```python
from build123d import *

# Parameters (mm, degrees)
BOX001_W        = 35
BOX001_H        = 47
BOX001_DEPTH    = 4
SKETCH006_W     = 6.802042
SKETCH006_H     = 4
PAD003_DEPTH    = 14
SKETCH007_R     = 1.647159
SKETCH007_R_2   = 1.531135
POCKET003_DEPTH = 7
PAD004_DEPTH    = 4
SKETCH009_R     = 4.5
SKETCH009_R_2   = 1.7
POCKET004_DEPTH = 4


with BuildPart() as part:
    # Box001 → Box001 (new body)
    with BuildSketch(Plane(origin=(-11, -31, -17), x_dir=(1, 0, 0), z_dir=(0, 0, 1))):
        with Locations((17.5, 23.5)):
            Rectangle(BOX001_W, BOX001_H)
    extrude(amount=BOX001_DEPTH)

    # Sketch006 → Pad003 (new body)
    with BuildSketch(Plane(origin=(-11, -31, -17), x_dir=(1, 0, 0), z_dir=(0, 0, -1))):
        with Locations((9.901021, -9.91944)):
            Rectangle(SKETCH006_W, SKETCH006_H)
        with Locations((9.901021, -37.91944)):
            Rectangle(SKETCH006_W, SKETCH006_H)
    extrude(amount=PAD003_DEPTH)

    # Sketch007 → Pocket003 (cut)
    with BuildSketch(Plane(origin=(2.302042, -31, -17), x_dir=(0, 1, 0), z_dir=(1, 0, 0))):
        with Locations((9.935232, -7.037912)):
            Circle(SKETCH007_R)
        with Locations((37.888477, -7.037912)):
            Circle(SKETCH007_R_2)
    extrude(amount=-POCKET003_DEPTH, mode=Mode.SUBTRACT)

    # Sketch008 → Pad004 (new body)
    with BuildSketch(Plane(origin=(-11, -31, -17), x_dir=(1, 0, 0), z_dir=(0, 0, -1))):
        with BuildLine():
            ThreePointArc((35, -34.9498), (43.145898, -23.9498), (35, -12.9498))
            Line((35, -12.9498), (35, -34.9498))
        make_face()
        with BuildLine():
            ThreePointArc((0, -12.9498), (-8.145898, -23.9498), (0, -34.9498))
            Line((0, -12.9498), (0, -34.9498))
        make_face()
    extrude(amount=-PAD004_DEPTH)

    # Sketch009 → Pocket004 (cut)
    with BuildSketch(Plane(origin=(-11, -31, -13), x_dir=(1, 0, 0), z_dir=(0, 0, 1))):
        with Locations((17.5, 38.5843)):
            Circle(SKETCH009_R)
        with Locations((-5.645898, 23.9498)):
            Circle(SKETCH009_R_2)
        with Locations((40.645898, 23.9498)):
            Circle(SKETCH009_R_2)
    extrude(amount=-POCKET004_DEPTH, mode=Mode.SUBTRACT)


solid = part.part
```
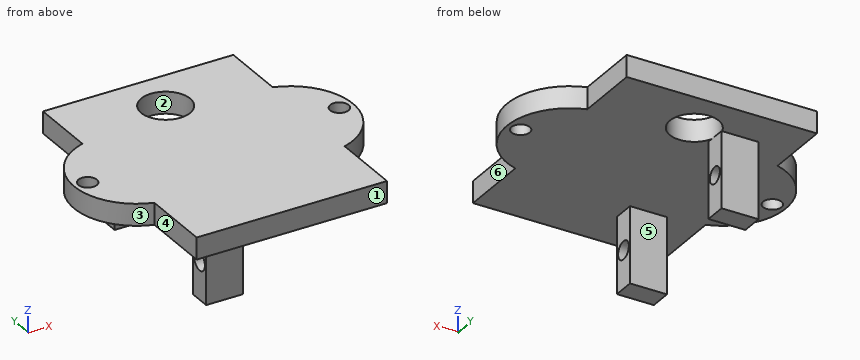
Source: CAD feature listing. Evaluate the final solid. Frame: model axes, mm. Face numbers are marked on the shaded views. A direction names the side the tool comes from. Round coordinates to 2 decimals unless told otherwise and drop trailing zeros. Loops run counter-clockwise (first coordinate to the right, second up) from the corner with the lowest first, then second, coordinate; pieces in that order, holes last. Notation, with made-up numbers: M -38,63 L -20,63 A17 cw -20,88 Z; hole C 80.25,58.25 d3. An arc over 180 degrees is marked long. Put each result on its own line as item: value.
(1) Section C-C, the plane y = -8. Return loops of the section in (x, z), and give its area (3 significant figures).
Solutions:
outline: M -19.11,-17 L -18.06,-17 L -18.06,-13 L -19.11,-13 Z; M -15.24,-17 L 28.24,-17 L 28.24,-13 L -15.24,-13 Z; M 31.06,-17 L 32.11,-17 L 32.11,-13 L 31.06,-13 Z
area: 182 mm²
(2) Pull-direction query (X, two-part tool) for the marked faces 1, 2 and 3; classes: released by +X, released by -X, zero draft, split by the parting line, or undercut.
Solutions:
face 1: zero draft
face 2: undercut
face 3: released by -X
(3) Access query for the marked faces 4, 5 and 6. Directions: +Z, -Z, +X, -X, +Y, -Y. A direction counts if a zero-diameter tool reaches every point of the face in a straight line with its end or side. Return the directions, or none.
Solutions:
face 4: +Z, -Z, -X, -Y
face 5: -Z, +X, -X
face 6: +Z, -Z, +X, -Y
(4) Section B-B, the plane z = -29.5. Return loops of the section in (x, y).
Solutions:
outline: M -4.5,-23.08 L 2.3,-23.08 L 2.3,-19.08 L -4.5,-19.08 Z; M -4.5,4.92 L 2.3,4.92 L 2.3,8.92 L -4.5,8.92 Z
(5) Section A-A, the plane x = 6.5. Return loops of the section in (y, z).
Solutions:
outline: M -31,-17 L 3.08,-17 L 3.08,-13 L -31,-13 Z; M 12.08,-17 L 16,-17 L 16,-13 L 12.08,-13 Z
(6) Ray query, line 1 (Y direction, x = -1, z = -17.5); line 2 (Z direction, x = 24, y = -13.5); line 3 (X direction, y = -24.5, z = -16.5). Return the intervals inside material, ascending. Write a range as [from, to].
Solutions:
line 1: [-23.08, -19.08], [4.92, 8.92]
line 2: [-17, -13]
line 3: [-11, 24]
(7) First-contact query: pin 1 (4.5 mm diameter, centred on y = 6.5, z = -27.5, fed in from -X); pin 2 (8 mm diameter, centred on y = -15.5, z = -17, fed in from +X); pin 3 (1.5 mm diameter, centred on y = -9.5, z = -15, fed in from +X). Flat tips, straight axial feed; report the tip coordinate or a pass-through.
Solutions:
pin 1: x = -4.5
pin 2: x = 31.25
pin 3: x = 32.02
(8) Section D-D, the plane x = 20. Return loops of the section in (y, z).
Solutions:
outline: M -31,-17 L 16,-17 L 16,-13 L -31,-13 Z
